```python
from build123d import *

# Parameters (mm, degrees)
SKETCH1_R           = 1.651
BOSS_EXTRUDE1_DEPTH = 6.35
SKETCH2_W           = 12.7
SKETCH2_H           = 3.175
CUT_EXTRUDE7_DEPTH  = 8.89
FILLET2_R           = 1.27
SKETCH4_W           = 3.175
SKETCH4_H           = 19.05
CUT_EXTRUDE8_DEPTH  = 192.82600491
FILLET3_R           = 1.27
SKETCH5_R           = 2.8575
SKETCH5_R_2         = 3.175
CUT_EXTRUDE9_DEPTH  = 2.54


with BuildPart() as part:
    # Sketch1 → Boss-Extrude1 (new body)
    with BuildSketch(Plane(origin=(0, 0, 0), x_dir=(1, 0, 0), z_dir=(0, 1, 0))):
        Polygon((75.155177047, 61.997896552), (75.155177047, 11.997896552), (91.919177047, 11.997896552), (91.919177047, 20.379896552), (83.537177047, 20.379896552), (83.537177047, 53.615896552), (173.037829354, 53.615896552), (173.037829354, 20.379896552), (164.655829354, 20.379896552), (164.655829354, 11.997896552), (181.419829354, 11.997896552), (181.419829354, 61.997896552), align=None)
        with Locations(Location((80.3721812, 16.064784874, 0), (0, 0, 270))):
            Circle(SKETCH1_R, mode=Mode.SUBTRACT)
        with Locations(Location((80.3721812, 57.93100823, 0), (0, 0, 270))):
            Circle(SKETCH1_R, mode=Mode.SUBTRACT)
        with Locations(Location((88.7874552, 16.064784874, 0), (0, 0, 270))):
            Circle(SKETCH1_R, mode=Mode.SUBTRACT)
        with Locations(Location((167.7875512, 57.93100823, 0), (0, 0, 270))):
            Circle(SKETCH1_R, mode=Mode.SUBTRACT)
        with Locations(Location((88.7874552, 57.93100823, 0), (0, 0, 270))):
            Circle(SKETCH1_R, mode=Mode.SUBTRACT)
        with Locations(Location((176.2028252, 57.93100823, 0), (0, 0, 270))):
            Circle(SKETCH1_R, mode=Mode.SUBTRACT)
        with Locations(Location((176.2028252, 16.064784874, 0), (0, 0, 270))):
            Circle(SKETCH1_R, mode=Mode.SUBTRACT)
        with Locations(Location((167.7875512, 16.064784874, 0), (0, 0, 270))):
            Circle(SKETCH1_R, mode=Mode.SUBTRACT)
    extrude(amount=BOSS_EXTRUDE1_DEPTH)

    # Sketch2 → Cut-Extrude7 (cut)
    with BuildSketch(Plane(origin=(181.419829354, 0, 0), x_dir=(0, 0, -1), z_dir=(1, 0, 0))):
        with Locations((43.747896552, 4.7625)):
            Rectangle(SKETCH2_W, SKETCH2_H)
    extrude(amount=-CUT_EXTRUDE7_DEPTH, mode=Mode.SUBTRACT)

    # Fillet2
    fillet2_edges = [part.edges().sort_by_distance(p)[0] for p in [
        (177.228829354, 6.35, -37.397896552),
        (177.228829354, 6.35, -50.097896552),
        (177.228829354, 3.175, -50.097896552),
        (177.228829354, 3.175, -37.397896552),
    ]]
    fillet(fillet2_edges, radius=FILLET2_R)

    # Sketch4 → Cut-Extrude8 (cut, through all)
    with BuildSketch(Plane(origin=(0, 6.35, 0), x_dir=(1, 0, 0), z_dir=(0, 1, 0))):
        with Locations((81.949677047, 29.904896552)):
            Rectangle(SKETCH4_W, SKETCH4_H)
    extrude(amount=-CUT_EXTRUDE8_DEPTH, mode=Mode.SUBTRACT)

    # Fillet3
    fillet3_edges = [part.edges().sort_by_distance(p)[0] for p in [
        (83.537177047, 3.175, -39.429896552),
        (80.362177047, 3.175, -20.379896552),
        (80.362177047, 3.175, -39.429896552),
    ]]
    fillet(fillet3_edges, radius=FILLET3_R)

    # Sketch5 → Cut-Extrude9 (cut)
    with BuildSketch(Plane.XZ):
        with Locations(Location((88.7874552, -16.064784874, 0), (0, 0, 270))):
            Circle(SKETCH5_R)
        with Locations(Location((88.7874552, -57.93100823, 0), (0, 0, 270))):
            Circle(SKETCH5_R_2)
        with Locations(Location((167.7875512, -57.93100823, 0), (0, 0, 270))):
            Circle(SKETCH5_R_2)
        with Locations(Location((167.7875512, -16.064784874, 0), (0, 0, 270))):
            Circle(SKETCH5_R)
    extrude(amount=-CUT_EXTRUDE9_DEPTH, mode=Mode.SUBTRACT)


solid = part.part
```
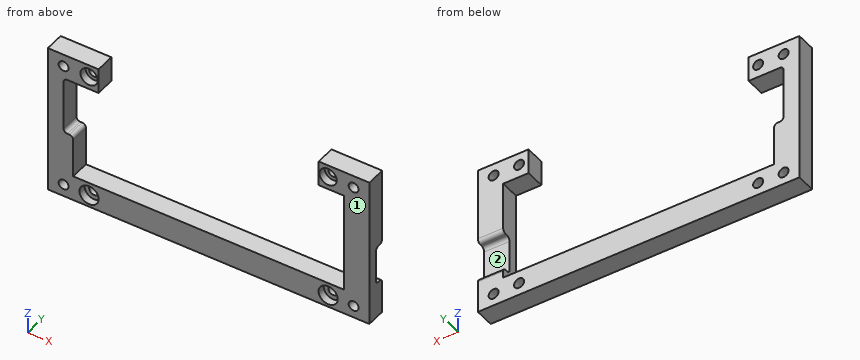
For this review, take the finished solid that the model builds, in its own axes (mm). Face numbers are marked on the shaded views. A direction names the side the tool comes from. Coordinates: 2 decimals unless noted, no trailing zeros. Write each loop counter-clockwise with the first axis right and the second up, starting at its lowest first coordinate (ties: lowest second). Pieces come first, ordered by that corner, then holes.
(1) Add section B-B on y = 1.5. Count the separate pieces of the cut face and the enclosed holes in it, then the cut area to 3 significant figures.
(2) For pin 1 Ø5.5 at (x, z) = (167.79, -57.93) entering from -Y; pin 2 Ø2.5 at (x, z) = (176.2, -57.93) entering from -Y; pin 3 Ø4 at (x, z) = (177, -45) entering from +Y (3 decimals), all flat-tipped, find the tip position at first contact; note any pin that passes through.
(3) Tool access review of the marked faces 1 and 2: name each direction out of +Z, -Z, +X, -X, +Y, -Y from which nothing blocks a thin tool from reaching the whole face with its end or side.
(4) Add section A-A on z = -23.5. Give the boundary of the cut face in (x, y), then the cut area to 3 significant figures.
(5) Add section C-C on x = 138.5. Give the boundary of the cut face in (y, z).
(6) Wall thickness on probe 1 along Z at (x, y) = (89, 3); probe 2 along Z at (x, y) = (167.5, 2); probe 3 along X at (y, z) = (1.75, -27.5): over which ranges is each line inside the solid? List them lowest first.
Answer sheet:
1. separate pieces: 1
1. enclosed holes: 8
1. area: 1,520 mm2
2. pin 1: stops at y = 2.54
2. pin 2: passes through
2. pin 3: stops at y = 3.175
3. face 1: +Z, -Z, +X, -X, -Y
3. face 2: +X, +Y
4. outline: (75.16, 0) - (80.36, 0) - (80.36, 6.35) - (75.16, 6.35) - close; (173.04, 0) - (181.42, 0) - (181.42, 6.35) - (173.04, 6.35) - close
4. area: 86.3 mm2
5. outline: (0, -62) - (6.35, -62) - (6.35, -53.62) - (0, -53.62) - close
6. probe 1: z = -62 to -59.57, -56.29 to -53.62, -20.38 to -17.7, -14.43 to -12
6. probe 2: z = -62 to -61.09, -54.77 to -53.62, -20.38 to -18.91, -13.22 to -12
6. probe 3: x = 75.16 to 80.36, 173.04 to 181.42
